Geometry: final body of the model. Coordinates: model frame, mm. A direction names the side the tool comes from. Give positions to 0.01 mm unless a question says otherwise; leave off trailing zeros. Write each loop counter-clockwise with the first axis right and the second up, starting at its lowest first coordinate (ties: lowest second). Pieces come first, ordered by that corner, then holes.
```python
from build123d import *

# Parameters (mm, degrees)
BOSS_EXTRUDE5_DEPTH     = 10
BOSS_EXTRUDE6_DEPTH     = 210
CUT_EXTRUDE1_DEPTH      = 577.072414333
CUT_EXTRUDE1_DEPTH_BACK = 577.072414333
SKETCH6_R               = 19.05


with BuildPart() as part:
    # Sketch1 → Boss-Extrude5 (new body)
    with BuildSketch(Plane(origin=(0, 0, 0), x_dir=(1, 0, 0), z_dir=(0, 1, 0))):
        Polygon((-69.524052506, -40.777590524), (-69.524052506, 249.222409476), (-39.524052506, 249.222409476), (24.115557801, 185.58279917), (24.115557801, 105.58279917), (59.115557801, 105.58279917), (59.115557801, 185.58279917), (122.755168108, 249.222409476), (186.394778415, 185.58279917), (186.394778415, 105.58279917), (221.394778415, 105.58279917), (221.394778415, 185.58279917), (283.247626246, 247.435647001), (346.887236552, 183.796036694), (346.887236552, 105.58279917), (381.887236552, 105.58279917), (381.887236552, 185.58279917), (445.526846859, 249.222409476), (470.475947494, 249.222409476), (470.475947494, -40.777590524), align=None)
    extrude(amount=BOSS_EXTRUDE5_DEPTH)

    # Sketch5 → Boss-Extrude6 (add)
    with BuildSketch(Plane(origin=(0, 10, 0), x_dir=(1, 0, 0), z_dir=(0, 1, 0))):
        Polygon((-69.524052506, -40.777590524), (-69.524052506, 249.222409476), (-63.174052506, 249.222409476), (-63.174052506, -34.427590524), (464.125947494, -34.427590524), (464.125947494, 249.222409476), (470.475947494, 249.222409476), (470.475947494, -40.777590524), align=None)
    extrude(amount=BOSS_EXTRUDE6_DEPTH)

    # Sketch6 → Cut-Extrude1 (cut, two sides: drawn at the far end of the back side and taken through both)
    with BuildSketch(Plane.XY.offset(-CUT_EXTRUDE1_DEPTH_BACK)):
        with Locations((200.475947494, 70)):
            Circle(SKETCH6_R)
    extrude(amount=CUT_EXTRUDE1_DEPTH + CUT_EXTRUDE1_DEPTH_BACK, mode=Mode.SUBTRACT)


solid = part.part
```
Item 1: Line query: L1, parallel to X at y = 198.5, z = -104.5; L2, parallel to X at y = 70, z = 36; L3, parallel to Z at x = 138.5, y = 187.5. Output: solid intervals per line, ascending.
Found:
L1: x = -69.52 to -63.17, 464.13 to 470.48
L2: x = -69.52 to 181.43, 219.53 to 470.48
L3: z = 34.43 to 40.78
Item 2: Reachability of faces 5 (the face through (59.116, 5, -145)), 6 (the face through (466, 101, -249.222)), 7 (the face through (-63.174, 114, -109)) from +Z, -Z, +X, -X, +Y, -Y: full face, straight path, thin tool, end or side. Return the list, or none.
Found:
face 5: -Z, +Y, -Y
face 6: -Z, +X, -X, +Y, -Y
face 7: -Z, +Y
Item 3: Section B-B, the plane y = 167. Return the cut outline in (x, z), plus the area to 3 significant figures.
Found:
outline: (-69.52, -249.22) - (-63.17, -249.22) - (-63.17, 34.43) - (464.13, 34.43) - (464.13, -249.22) - (470.48, -249.22) - (470.48, 40.78) - (-69.52, 40.78) - close
area: 7,030 mm2
Item 4: Section C-C, the plane z = -19. Return the cut outline in (x, y), plus the area to 3 significant figures.
Found:
outline: (-69.52, 0) - (470.48, 0) - (470.48, 220) - (464.13, 220) - (464.13, 10) - (-63.17, 10) - (-63.17, 220) - (-69.52, 220) - close
area: 8,070 mm2
Item 5: Pin query (flat end, axial travel): pin 1 Ø11 at (x, y) = (40, 6.5) entering from -Z; pin 2 Ø8 at (x, y) = (174, 190.5) entering from -Z; pin 3 Ø2 at (x, z) = (396, -161) entering from +Y. Return the tip coordinate at first contact, or that it passes through.
Found:
pin 1: stops at z = -105.58
pin 2: stops at z = 34.43
pin 3: stops at y = 10
Item 6: Section D-D, the plane x = 425. Return the cut outline in (y, z).
Found:
outline: (0, -228.7) - (10, -228.7) - (10, 34.43) - (220, 34.43) - (220, 40.78) - (0, 40.78) - close
Item 7: Section A-A, the plane y = 70. Return the cut outline in (x, z).
Found:
outline: (-69.52, -249.22) - (-63.17, -249.22) - (-63.17, 34.43) - (181.43, 34.43) - (181.43, 40.78) - (-69.52, 40.78) - close; (219.53, 34.43) - (464.13, 34.43) - (464.13, -249.22) - (470.48, -249.22) - (470.48, 40.78) - (219.53, 40.78) - close
Item 8: Pull-direction query (X, two-part tool) for faces 1 (the face through (413.262, 4.93, -216.957)), 2 (the face through (186.395, 5, -146)), 3 (the face through (-69.524, 108, -102)), 4 (the face through (202, 220, 35)); classes: +X half, -X half, draft (parallel to the pull), parting line (faces both ways), or undercut.
Found:
face 1: undercut
face 2: undercut
face 3: -X half
face 4: draft
